Work out the finished part from the listing and answer in its coordinate system (mm). A direction names the side the tool comes from. Round coordinates to 2 decimals unless told otherwise and drop trailing zeros. Order: outer loops, then holes, each group sorted by start corner. A loop starts at its lowest first (then second) coordinate and runs counter-clockwise, first axis right, second up. Notation, with made-up numbers: (8, -5.5) - (32, -5.5) arc R23 cw to (32, 22.5) - close; hole circle Ø9 at (-4, -3.75). An arc over 180 degrees is marked (long way). Put each result on its own line as item: value.
```python
from build123d import *

# Parameters (mm, degrees)
F0_W             = 12.5
F0_H             = 25
F1_DEPTH         = 10.16
F2_W             = 7.112
F2_H             = 6.35
F3_DEPTH         = 25.4
F4_W             = 1.27
F4_H             = 1.27
F5_DEPTH         = 10.16
F5_COPIES2_COUNT = 2
F5_COPIES2_PITCH = 20.028927
F8_DEPTH         = 25.4


# Not quite as in the source:
# - a pattern or mirror of a feature is missing from the dataset's text; its kind, count and spacing are read off the source's solid


with BuildPart() as f1:
    # F0 (on Top) → F1 (new body)
    with BuildSketch(Plane.XY):
        Rectangle(F0_W, F0_H)
    extrude(amount=F1_DEPTH)

    # F2 (on face) → F3 (cut)
    with BuildSketch(Plane.XY.offset(10.16)):
        with Locations((0, -9.325)):
            Rectangle(F2_W, F2_H)
    f3 = extrude(amount=-F3_DEPTH, mode=Mode.SUBTRACT)

    # F3_copies: F3 across plane
    add(f3.mirror(Plane.ZX), mode=Mode.SUBTRACT)

    # F4 (on face) → F5 (join, through all)
    with BuildSketch(Plane.XY.offset(10.16)):
        with Locations((-2.921, -9.579)):
            Rectangle(F4_W, F4_H)
    f5 = extrude(amount=-F5_DEPTH)

    # F5_copies: F5 across plane
    add(f5.mirror(Plane(origin=(0, 0, 0), x_dir=(0, 0, 1), z_dir=(1, 0, 0))))

    # F5_copies1: F5 across plane
    add(f5.mirror(Plane.ZX))

    # F5_copies2: F5 ×2
    with Locations(*[Vector(0.2916781273, 0.9565165289, 0) * (i * F5_COPIES2_PITCH) for i in range(1, F5_COPIES2_COUNT)]):
        add(f5)

    # F7 (on face) → F8 (cut)
    with BuildSketch(Plane.XY.offset(10.16)):
        Polygon((-0.8082230509, 0.8082230509), (-4.5205336521, -2.9040875503), (-3.7123106012, -3.7123106012), (0, 0), align=None)
        Polygon((2.9040875503, 4.5205336521), (-0.8082230509, 0.8082230509), (0, 0), (-3.7123106012, -3.7123106012), (-2.9040875503, -4.5205336521), (4.5205336521, 2.9040875503), align=None)
    f8 = extrude(amount=-F8_DEPTH, mode=Mode.SUBTRACT)

    # F8_copies: F8 across plane
    add(f8.mirror(Plane(origin=(0, 0, 0), x_dir=(0, 0, 1), z_dir=(1, 0, 0))), mode=Mode.SUBTRACT)


solid = f1.part
```
1) A cutting plane is placed at D-D on y = -2.25. Write down the section's boundary in (x, z), then the cut area to 3 significant figures.
Findings below:
outline: (-6.25, 0) - (-3.87, 0) - (-3.87, 10.16) - (-6.25, 10.16) - close; (-0.63, 0) - (0.63, 0) - (0.63, 10.16) - (-0.63, 10.16) - close; (3.87, 0) - (6.25, 0) - (6.25, 10.16) - (3.87, 10.16) - close
area: 61.3 mm2
2) A cutting plane is placed at A-A on y = 7.25. Write down the section's boundary in (x, z), then the cut area to 3 significant figures.
Findings below:
outline: (-6.25, 0) - (-3.56, 0) - (-3.56, 10.16) - (-6.25, 10.16) - close; (3.56, 0) - (6.25, 0) - (6.25, 10.16) - (3.56, 10.16) - close
area: 54.7 mm2
3) Straight lines are drawn through the part: L1, parallel to X at y = -7, z = 2.25; L2, parallel to Y at x = 2.75, z = 5.5; L3, parallel to Y at x = 2, z = 9. For each, find the intervals that lie inside material, in ascending order. Write a range as from..to.
Findings below:
L1: x = -6.25..-3.56, 3.56..6.25
L2: y = -10.21..-8.94, -6.15..-4.37, -1.13..1.13, 4.37..6.15, 8.94..10.21
L3: y = -6.15..-3.62, -0.38..0.38, 3.62..6.15
4) Given pin 1 Ø5.5 at (x, z) = (0, 3.5) entering from +Y; pin 2 Ø0.6 at (x, z) = (-3, 5) entering from -Y, each flat-ended and moving along its own axis, determine where each tip first touches the part or whether it passes through.
Findings below:
pin 1: stops at y = 10.21
pin 2: stops at y = -10.21
5) For faces 1 (the flat face through (-3, 10.214, 5)), 2 (the flat face through (3, -10.214, 5)), 3 (the flat face through (-3, 0, 10.16)), 4 (the flat face through (3.048, 1.432, 5.151)), determine the directions among +Z, -Z, +X, -X, +Y, -Y from which every point of the face is accessible in a straight line to the end or side of a thin tool.
Findings below:
face 1: +Z, -Z, +Y
face 2: +Z, -Z, -Y
face 3: +Z, +X, -X, +Y, -Y
face 4: +Z, -Z
6) A cutting plane is placed at B-B on x = 1. Write down the section's boundary in (y, z).
Findings below:
outline: (-6.15, 0) - (-2.62, 0) - (-2.62, 10.16) - (-6.15, 10.16) - close; (2.62, 0) - (6.15, 0) - (6.15, 10.16) - (2.62, 10.16) - close
7) A cutting plane is placed at C-C on y = 3.75. Write down the section's boundary in (x, z).
Findings below:
outline: (-6.25, 0) - (-3.67, 0) - (-3.67, 10.16) - (-6.25, 10.16) - close; (-2.13, 0) - (2.13, 0) - (2.13, 10.16) - (-2.13, 10.16) - close; (3.67, 0) - (6.25, 0) - (6.25, 10.16) - (3.67, 10.16) - close
8) For a pull along Y with two mould halves and no side action, classify faces 5 (the flat face through (-2.286, 10, 5)), 6 (the flat face through (0, 6.15, 5)), 7 (the flat face through (-3, -10.214, 5)), 8 (the flat face through (3.048, -1.432, 5.151)) as pulls with the +Y half, pulls with the -Y half, needs draft (parallel to the pull), parting line crosses it, or undercut.
Findings below:
face 5: needs draft
face 6: undercut
face 7: pulls with the -Y half
face 8: undercut
